Autodesk Fusion 360 part; units mm, degrees
sketch "Sketch1" plane through (0, 0, 0) normal (0, 0, 1) x (1, 0, 0)
  circle A0 centre (0, 0) radius 6.35
  dimension "d1" = 12.7
extrude "Extrude1" add sketch "Sketch1" along normal blind 25.4
ref_plane "WorkPlane1" through (0, -6.35, 16.0163) normal (0, -1, 0) x (-1, 0, 0)
sketch "Sketch2" plane through (0, -6.35, 16.0163) normal (0, -1, 0) x (1, 0, 0)
  line L0 (6.35, 9.3837) -> (-6.35, 9.3837)
  line L1 (6.35, -16.0163) -> (-6.35, -16.0163)
  point P0 (0, 9.3837)
ref_plane "WorkPlane2" through (0, 0, 22.225) normal (0, 0, 1) x (1, 0, 0)
sketch "Sketch4" plane through (0, 0, 22.225) normal (0, 0, 1) x (1, 0, 0)
  circle A0 centre (0, 0) radius 6.35
  line L0 (0, 0) -> (0, -6.35) construction
  line L1 (0, 0) -> (5.4993, 3.175) construction
  line L2 (0, 0) -> (-5.4993, 3.175) construction
  dimension "d22" = 360
hole "Hole1" at (0, -6.35, 25.4) direction (0, 1, 0) diameter 6.35 depth 6.35 tip angle 180
pattern_circular "C-Pattern1" count 3 over 360 about axis through (0, 0, 0) along (0, 0, 1) of "Hole1"
extrude "Extrude2" cut sketch "Sketch4" against normal blind 0.127 from surface at 3.175
hole "Hole2" at (0, 0, 0) direction (0, 0, 1) diameter 2.2708 depth 12.573 tip angle 180
hole "Hole3" at (0, 0, 0) direction (0, 0, 1) diameter 5.1181 depth 19.05 tip angle 180
equation "d5 = d1 / 2"
Geometry check sheet. Reference: the model listing, model coordinates, mm. A direction names the side the tool comes from. Coordinates: 2 decimals unless noted, no trailing zeros. Order: outer loops, then holes, each group sorted by start corner. A loop starts at its lowest first (then second) coordinate and runs counter-clockwise, first axis right, second up. Notation, with made-up numbers: (11, 65.5) -> (52, 65.5) arc R21 ccw to (52, 95.5) -> close; hole circle Ø4 at (-3, -11.5). An arc over 180 degrees is marked (long way). Use a Markdown table: item, result. Add a question column.
1. Cross-section at C-C (z = 19.5). Enter the section's corners in (x, y), and give its area (3 significant figures).
2. Set-up check for faces 4 (the face through (3, 0, 0)), 5 (the face through (0.63, 1.09, 24.11)), 6 (the face through (-0.113, -2.557, 9.658)): record each of +Z, -Z, +X, -X, +Y, -Y from which the full face is reachable in a straight line by a thin tool's end or side.
3. Cross-section at B-B (z = 9). Enter the section's corners in (x, y).
4. Cross-section at D-D (y = -3.25). Enter the section's corners in (x, z) (3 decimals), and give its area (3 significant figures).
5. Cross-section at A-A (x = 2). Enter the section's corners in (y, z).
6. Go/stop test with flat-tipped pins: pin 1 Ø4 at (y, z) = (3.5, 4) entering from -X; pin 2 Ø4.5 at (x, y) = (0, 0) entering from -Z; pin 3 Ø2 at (x, z) = (2, 16) entering from +Y. Record where each tip stops, or that it passes through.
7. Mould release check, pull along Y, two halves, no side actions. Record for faces 1 (the face through (-2.745, 1.506, 22.226)), 2 (the face through (1, 0, 24)), 3 (the face through (0.068, -3.131, 22.226)): pulls with the +Y half, pulls with the -Y half, needs draft (parallel to the pull), parting line crosses it, or undercut.
8. Material ranges on L1, parallel to Y at x = 0, z = 15.25; L2, parallel to Y at x = -5.5, z = 16.5, recorded low to high.
Filled sheet:
| question | item | result |
|---|---|---|
| 1 | outline | circle Ø12.7 at (0, 0) |
| 1 | area | 127 mm2 |
| 2 | face 4 | -Z, +X, -X, +Y, -Y |
| 2 | face 5 | +Z |
| 2 | face 6 | -Z |
| 3 | outline | circle Ø12.7 at (0, 0); hole circle Ø5.12 at (0, 0) |
| 4 | outline | (-5.455, 0) -> (5.455, 0) -> (5.455, 25.273) -> (3.172, 25.273) arc R3.175 cw to (-3.172, 25.273) -> (-5.455, 25.273) -> close |
| 4 | area | 261 mm2 |
| 5 | outline | (-6.03, 0) -> (-1.6, 0) -> (-1.6, 19.05) -> (1.6, 19.05) -> (1.6, 0) -> (6.03, 0) -> (6.03, 25.27) -> (0, 25.27) -> (0, 22.93) -> (-6.03, 22.93) -> close |
| 6 | pin 1 | x = -6.17 |
| 6 | pin 2 | z = 19.05 |
| 6 | pin 3 | y = 6.27 |
| 7 | face 1 | undercut |
| 7 | face 2 | pulls with the -Y half |
| 7 | face 3 | needs draft |
| 8 | L1 | -6.35 to -2.56, 2.56 to 6.35 |
| 8 | L2 | -3.17 to 3.17 |
